The listing builds one solid part. Answer for the finished solid, in the listing's coordinates (mm). Give positions to 0.01 mm unless a question says otherwise; leave off trailing zeros. Write each loop counter-clockwise with the first axis right and the second up, starting at its lowest first coordinate (ties: lowest second). Pieces come first, ordered by that corner, then holes. Notation, with made-up numbers: (73, 51) -> (116, 51) arc R22 ccw to (116, 72) -> close; hole circle Ø5 at (-38, 61.25). An arc over 180 degrees is marked (long way). One line per question, with ' | ' between items.
from build123d import *

# Parameters (mm, degrees)
F0_R     = 11.25
F1_DEPTH = 7
F2_SIZE  = 1.99999


# Not quite as in the source:
# - a fillet or chamfer is up to 0.001 mm smaller than in the source, because OpenCascade refuses the exact size
# - a feature names something its author has since deleted; it is built from what else it names


with BuildPart() as f1:
    # F0 (on Top) → F1 (new body)
    with BuildSketch(Plane.XY):
        with BuildLine():
            ThreePointArc((32.9748366001, -13.25), (44.4496732003, -6.625), (44.4496732003, 6.625))
            ThreePointArc((44.4496732003, 6.625), (35.3296022004, 13.0390789156), (24.5421176937, 10.2201639833))
            ThreePointArc((24.5421176937, 10.2201639833), (22.9496732003, 19.0380307876), (16.1093987873, 24.8260615752))
            ThreePointArc((16.1093987873, 24.8260615752), (23.9443929832, 32.7588397347), (22.9496732003, 43.8640923627))
            ThreePointArc((22.9496732003, 43.8640923627), (11.4748366001, 50.4890923627), (0, 43.8640923627))
            ThreePointArc((0, 43.8640923627), (-1.6185408213, 35.2078445445), (2.5465871703, 27.4488491524))
            ThreePointArc((2.5465871703, 27.4488491524), (4.5677953806, 25.931781383), (6.840274413, 24.8260615752))
            ThreePointArc((6.840274413, 24.8260615752), (0, 19.0380307876), (-1.5924444934, 10.2201639833))
            ThreePointArc((-1.5924444934, 10.2201639833), (-12.3799290001, 13.0390789156), (-21.5, 6.625))
            ThreePointArc((-21.5, 6.625), (-21.5, -6.625), (-10.0251633999, -13.25))
            ThreePointArc((-10.0251633999, -13.25), (0.0896273829, -8.5588262876), (3.0421176937, 2.1928668043))
            ThreePointArc((3.0421176937, 2.1928668043), (11.4748366001, -0.8369692124), (19.9075555066, 2.1928668043))
            ThreePointArc((19.9075555066, 2.1928668043), (22.8600458174, -8.5588262876), (32.9748366001, -13.25))
        make_face()
        with BuildLine():
            ThreePointArc((-19.7679491924, 5.625), (-7.1134491425, 10.8666655458), (1.2248366001, 0))
            ThreePointArc((1.2248366001, 0), (-2.0702121115, -7.9549512883), (-10.0251633999, -11.25))
            ThreePointArc((-10.0251633999, -11.25), (-19.7679491924, -5.625), (-19.7679491924, 5.625))
        make_face(mode=Mode.SUBTRACT)
        with BuildLine():
            ThreePointArc((44.2248366001, 0), (40.9297878885, -7.9549512883), (32.9748366001, -11.25))
            ThreePointArc((32.9748366001, -11.25), (23.2320508076, 5.625), (42.7176223927, 5.625))
            ThreePointArc((42.7176223927, 5.625), (43.8415021459, 2.9117142574), (44.2248366001, 0))
        make_face(mode=Mode.SUBTRACT)
        with Locations((11.4748366001, 12.4130307876)):
            Circle(F0_R, mode=Mode.SUBTRACT)
        with BuildLine():
            ThreePointArc((1.7320508076, 42.8640923627), (14.3865508575, 48.1057579085), (22.7248366001, 37.2390923627))
            ThreePointArc((22.7248366001, 37.2390923627), (8.5631223427, 26.372426817), (1.7320508076, 42.8640923627))
        make_face(mode=Mode.SUBTRACT)
        with BuildLine():
            ThreePointArc((2.5465871703, 27.4488491524), (-1.6185408213, 35.2078445445), (0, 43.8640923627))
            Line((0, 43.8640923627), (-21.5, 6.625))
            ThreePointArc((-21.5, 6.625), (-12.3799290001, 13.0390789156), (-1.5924444934, 10.2201639833))
            ThreePointArc((-1.5924444934, 10.2201639833), (0, 19.0380307876), (6.840274413, 24.8260615752))
            ThreePointArc((6.840274413, 24.8260615752), (4.5677953806, 25.931781383), (2.5465871703, 27.4488491524))
        make_face()
        with BuildLine():
            ThreePointArc((24.5421176937, 10.2201639833), (35.3296022004, 13.0390789156), (44.4496732003, 6.625))
            Line((44.4496732003, 6.625), (22.9496732003, 43.8640923627))
            ThreePointArc((22.9496732003, 43.8640923627), (23.9443929832, 32.7588397347), (16.1093987873, 24.8260615752))
            ThreePointArc((16.1093987873, 24.8260615752), (22.9496732003, 19.0380307876), (24.5421176937, 10.2201639833))
        make_face()
        with BuildLine():
            Line((-10.0251633999, -13.25), (32.9748366001, -13.25))
            ThreePointArc((32.9748366001, -13.25), (22.8600458174, -8.5588262876), (19.9075555066, 2.1928668043))
            ThreePointArc((19.9075555066, 2.1928668043), (11.4748366001, -0.8369692124), (3.0421176937, 2.1928668043))
            ThreePointArc((3.0421176937, 2.1928668043), (0.0896273829, -8.5588262876), (-10.0251633999, -13.25))
        make_face()
    extrude(amount=F1_DEPTH)

    # F2 (size 2 in the source; OpenCascade refuses exactly that, so slightly less here)
    f2_edges = [f1.edges().sort_by_distance(p)[0] for p in [
        (33.699673, 25.244546, 0),
        (44.449673, -6.625, 0),
        (11.474837, -13.25, 0),
        (-21.5, -6.625, 0),
        (-10.75, 25.244546, 0),
        (11.474837, 50.489092, 0),
        (-10.75, 25.244546, 7),
    ]]
    chamfer(f2_edges, length=F2_SIZE)


solid = f1.part
Item 1: Consider line 1 (Y direction, x = 21, z = 4.5); line 2 (X direction, y = 9, z = 0.75); line 3 (Y direction, x = 18.5, z = 0.5). Determine where each line is inside the solid, lowest interval first. Write a range as [from, to].
Answers below:
line 1: [-13.25, 6.43], [18.4, 31.25], [43.23, 46.45] | line 2: [-18.69, -16.78], [-3.28, 0.76], [22.19, 26.22], [39.72, 41.64] | line 3: [-11.75, 3.63], [21.2, 28.45], [46.03, 46.66]
Item 2: Find section B-B (y = 28.5). Write down the section's boundary in (x, z), then the cut area to 3 significant figures.
Answers below:
outline: (-8.87, 2) -> (-6.56, 0) -> (4.39, 0) -> (4.39, 7) -> (-6.56, 7) -> (-8.87, 5) -> close; (18.56, 0) -> (29.51, 0) -> (31.82, 2) -> (31.82, 5) -> (29.51, 7) -> (18.56, 7) -> close | area: 176 mm²
Item 3: Flat-ended cylindrical pins translate along their axes: pin 1 (3 mm diameter, centred on y = 12.5, z = 5.5, fed in from -X); pin 2 (2 mm diameter, centred on x = -9, z = 5.5, fed in from +Y); pin 3 (2 mm diameter, centred on y = 19, z = 1, fed in from +X). Find the tip coordinate at first contact, or state that the pin passes through.
Answers below:
pin 1: x = -18.92 | pin 2: y = 29.78 | pin 3: x = 37.44
Item 4: Find section A-A (x = -9). Write down the section's boundary in (y, z), then the cut area to 3 significant figures.
Answers below:
outline: (-13.25, 2) -> (-11.25, 0) -> (-11.2, 0) -> (-11.2, 7) -> (-11.25, 7) -> (-13.25, 5) -> close; (11.2, 0) -> (24.28, 0) -> (28.28, 2) -> (28.28, 5) -> (24.28, 7) -> (11.2, 7) -> close | area: 122 mm²
Item 5: Find section C-C (y = 9). Write down the section's boundary in (x, z).
Answers below:
outline: (-20.13, 2) -> (-17.82, 0) -> (-16.78, 0) -> (-16.78, 7) -> (-17.82, 7) -> (-20.13, 5) -> close; (-3.28, 0) -> (0.76, 0) -> (0.76, 7) -> (-3.28, 7) -> close; (22.19, 0) -> (26.22, 0) -> (26.22, 7) -> (22.19, 7) -> close; (39.72, 0) -> (40.77, 0) -> (43.08, 2) -> (43.08, 5) -> (40.77, 7) -> (39.72, 7) -> close
Item 6: Find section D-D (x = 17.5). Count the separate pieces of the cut face and the enclosed holes in it, then the cut area to 3 significant figures.
Answers below:
separate pieces: 3 | enclosed holes: 0 | area: 161 mm²
Item 7: Determine the mould class of faces 1 (the face through (16.666, 2.432, 3.451)), 2 (the face through (32.972, 24.477, 6.014)), 3 (the face through (42.91, -5.93, 6.68)) for opening direction Y: pulls with the +Y half, pulls with the -Y half, needs draft (parallel to the pull), parting line crosses it, or undercut.
Answers below:
face 1: undercut | face 2: pulls with the +Y half | face 3: parting line crosses it
